from build123d import *

# Parameters (mm, degrees)
CROQUIS3_W              = 30
CROQUIS3_H              = 29
SALIENTE_EXTRUIR1_DEPTH = 5
CROQUIS5_W              = 30
CROQUIS5_H              = 29
CROQUIS5_W_2            = 25.5
CROQUIS5_H_2            = 24.5
CORTAR_EXTRUIR1_DEPTH   = 2
CROQUIS9_W              = 25.5
CROQUIS9_H              = 2.25
SALIENTE_EXTRUIR2_DEPTH = 13.5
CROQUIS11_W             = 22
CROQUIS11_H             = 6
CORTAR_EXTRUIR3_DEPTH   = 3
CROQUIS12_W             = 25.5
CROQUIS12_H             = 3.5
SALIENTE_EXTRUIR3_DEPTH = 15
CROQUIS13_W             = 25.5
CROQUIS13_H             = 4
SALIENTE_EXTRUIR4_DEPTH = 20
REDONDEO3_R             = 5
CROQUIS14_R             = 1.5
CORTAR_EXTRUIR4_DEPTH   = 7
REDONDEO5_R             = 10
REDONDEO6_R             = 40
CROQUIS6_R              = 1
CORTAR_EXTRUIR5_DEPTH   = 5
CORTAR_EXTRUIR7_DEPTH   = 2
CROQUIS16_W             = 21.5
CROQUIS16_H             = 5
CORTAR_EXTRUIR8_DEPTH   = 2


with BuildPart() as part:
    # Croquis3 → Saliente-Extruir1 (new body)
    with BuildSketch(Plane.XY):
        Rectangle(CROQUIS3_W, CROQUIS3_H)
    extrude(amount=SALIENTE_EXTRUIR1_DEPTH)

    # Croquis5 → Cortar-Extruir1 (cut)
    with BuildSketch(Plane.XY.offset(5)):
        Rectangle(CROQUIS5_W, CROQUIS5_H)
        Rectangle(CROQUIS5_W_2, CROQUIS5_H_2, mode=Mode.SUBTRACT)
    extrude(amount=-CORTAR_EXTRUIR1_DEPTH, mode=Mode.SUBTRACT)

    # Croquis9 → Saliente-Extruir2 (add)
    with BuildSketch(Plane.XY.offset(3)):
        with Locations((0, -13.375)):
            Rectangle(CROQUIS9_W, CROQUIS9_H)
    extrude(amount=SALIENTE_EXTRUIR2_DEPTH)

    # Croquis11 → Cortar-Extruir3 (cut)
    with BuildSketch(Plane.XZ.offset(14.5)):
        with Locations((0, 7.6)):
            Rectangle(CROQUIS11_W, CROQUIS11_H)
    extrude(amount=-CORTAR_EXTRUIR3_DEPTH, mode=Mode.SUBTRACT)

    # Croquis12 → Saliente-Extruir3 (add)
    with BuildSketch(Plane.XZ.offset(14.5)):
        with Locations((0, 12.75)):
            Rectangle(CROQUIS12_W, CROQUIS12_H)
    extrude(amount=SALIENTE_EXTRUIR3_DEPTH)

    # Croquis13 → Saliente-Extruir4 (add)
    with BuildSketch(Plane(origin=(0, 0, 11), x_dir=(-1, 0, 0), z_dir=(0, 0, -1))):
        with Locations((0, -27.5)):
            Rectangle(CROQUIS13_W, CROQUIS13_H)
    extrude(amount=SALIENTE_EXTRUIR4_DEPTH)

    # Redondeo3
    redondeo3_edges = [part.edges().sort_by_distance(p)[0] for p in [
        (0, -29.5, 14.5),
    ]]
    fillet(redondeo3_edges, radius=REDONDEO3_R)

    # Croquis14 → Cortar-Extruir4 (cut)
    with BuildSketch(Plane.XZ.offset(29.5)):
        with Locations((0, -3)):
            Circle(CROQUIS14_R)
    extrude(amount=-CORTAR_EXTRUIR4_DEPTH, mode=Mode.SUBTRACT)

    # Redondeo5
    # the kernel refuses this fillet: 10 mm, written as the material it adds along each edge
    with BuildSketch(Plane(origin=(12.75, -14.5, 11), x_dir=(0, -1, 0), z_dir=(-1, 0, 0))) as redondeo5_piece_1_section:
        with BuildLine():
            CenterArc((REDONDEO5_R, -REDONDEO5_R), REDONDEO5_R, 90, 90)
            Line((0, -REDONDEO5_R), (0, 0))
            Line((0, 0), (REDONDEO5_R, 0))
        make_face()
    redondeo5_piece_1 = extrude(amount=50.5, mode=Mode.PRIVATE)
    redondeo5_piece_1 = split(redondeo5_piece_1, bisect_by=Plane(origin=(11, -14.5, 11), z_dir=(1, 0, 0)), keep=Keep.TOP, mode=Mode.PRIVATE)
    add(redondeo5_piece_1)
    with BuildSketch(Plane(origin=(37.75, -14.5, 11), x_dir=(0, -1, 0), z_dir=(-1, 0, 0))) as redondeo5_piece_2_section:
        with BuildLine():
            CenterArc((REDONDEO5_R, -REDONDEO5_R), REDONDEO5_R, 90, 90)
            Line((0, -REDONDEO5_R), (0, 0))
            Line((0, 0), (REDONDEO5_R, 0))
        make_face()
    redondeo5_piece_2 = extrude(amount=50.5, mode=Mode.PRIVATE)
    redondeo5_piece_2 = split(redondeo5_piece_2, bisect_by=Plane(origin=(11, -14.5, 11), z_dir=(-1, 0, 0)), keep=Keep.TOP, mode=Mode.PRIVATE)
    redondeo5_piece_2 = split(redondeo5_piece_2, bisect_by=Plane(origin=(37.75, -14.5, 10.6), z_dir=(0, 0, 1)), keep=Keep.TOP, mode=Mode.PRIVATE)
    add(redondeo5_piece_2)
    with BuildSketch(Plane(origin=(37.75, -14.5, 11), x_dir=(0, -1, 0), z_dir=(-1, 0, 0))) as redondeo5_piece_3_section:
        with BuildLine():
            CenterArc((REDONDEO5_R, -REDONDEO5_R), REDONDEO5_R, 90, 90)
            Line((0, -REDONDEO5_R), (0, 0))
            Line((0, 0), (REDONDEO5_R, 0))
        make_face()
    redondeo5_piece_3 = extrude(amount=75.5, mode=Mode.PRIVATE)
    redondeo5_piece_3 = split(redondeo5_piece_3, bisect_by=Plane(origin=(37.75, -14.5, 3), z_dir=(0, 0, -1)), keep=Keep.TOP, mode=Mode.PRIVATE)
    redondeo5_piece_3 = split(redondeo5_piece_3, bisect_by=Plane(origin=(15, -14.5, 11), z_dir=(-1, 0, 0)), keep=Keep.TOP, mode=Mode.PRIVATE)
    redondeo5_piece_3 = split(redondeo5_piece_3, bisect_by=Plane(origin=(-15, -14.5, 11), z_dir=(1, 0, 0)), keep=Keep.TOP, mode=Mode.PRIVATE)
    add(redondeo5_piece_3)
    with BuildSketch(Plane(origin=(37.75, -14.5, 11), x_dir=(0, -1, 0), z_dir=(-1, 0, 0))) as redondeo5_piece_4_section:
        with BuildLine():
            CenterArc((REDONDEO5_R, -REDONDEO5_R), REDONDEO5_R, 90, 90)
            Line((0, -REDONDEO5_R), (0, 0))
            Line((0, 0), (REDONDEO5_R, 0))
        make_face()
    redondeo5_piece_4 = extrude(amount=50.5, mode=Mode.PRIVATE)
    redondeo5_piece_4 = split(redondeo5_piece_4, bisect_by=Plane(origin=(11, -14.5, 11), z_dir=(-1, 0, 0)), keep=Keep.TOP, mode=Mode.PRIVATE)
    redondeo5_piece_4 = split(redondeo5_piece_4, bisect_by=Plane(origin=(37.75, -14.5, 4.6), z_dir=(0, 0, -1)), keep=Keep.TOP, mode=Mode.PRIVATE)
    add(redondeo5_piece_4)
    with BuildSketch(Plane(origin=(37.75, -14.5, 11), x_dir=(0, -1, 0), z_dir=(-1, 0, 0))) as redondeo5_piece_5_section:
        with BuildLine():
            CenterArc((REDONDEO5_R, -REDONDEO5_R), REDONDEO5_R, 90, 90)
            Line((0, -REDONDEO5_R), (0, 0))
            Line((0, 0), (REDONDEO5_R, 0))
        make_face()
    redondeo5_piece_5 = extrude(amount=50.5, mode=Mode.PRIVATE)
    redondeo5_piece_5 = split(redondeo5_piece_5, bisect_by=Plane(origin=(-11, -14.5, 11), z_dir=(-1, 0, 0)), keep=Keep.TOP, mode=Mode.PRIVATE)
    add(redondeo5_piece_5)
    with BuildSketch(Plane(origin=(-12.75, -14.5, 14.5), x_dir=(0, -1, 0), z_dir=(1, 0, 0))) as redondeo5_piece_6:
        with BuildLine():
            CenterArc((6, -10), REDONDEO5_R, 90, 36.869897646)
            Line((0, -2), (0, 0))
            Line((0, 0), (6, 0))
        make_face()
    extrude(amount=25.5)

    # Redondeo6
    # the kernel refuses this fillet: 40 mm, written as the material it adds along each edge
    with BuildSketch(Plane(origin=(-12.75, -25.5, 11), x_dir=(0, 1, 0), z_dir=(1, 0, 0))) as redondeo6_piece_1:
        with BuildLine():
            CenterArc((40, -8.888194417), REDONDEO6_R, 167.161431859, 12.838568141)
            Line((0, -8.888194417), (-0.8, -8.888194417))
            Line((-0.8, -8.888194417), (-0.8, 0))
            Line((-0.8, 0), (0, 0.8))
            ThreePointArc((0, 0.8), (0.5, 0.8), (0.22, 0.177763888))
            Line((0.22, 0.177763888), (1, 0))
        make_face()
    extrude(amount=25.5)

    # Croquis6 → Cortar-Extruir5 (cut)
    with BuildSketch(Plane.XY):
        with Locations((-10.75, 9.75)):
            Circle(CROQUIS6_R)
        with Locations((-10.75, -3.75)):
            Circle(CROQUIS6_R)
        with Locations(Location((10.75, -3.75, 0), (0, 0, 180))):
            Circle(CROQUIS6_R)
        with Locations(Location((10.75, 9.75, 0), (0, 0, 180))):
            Circle(CROQUIS6_R)
    extrude(amount=CORTAR_EXTRUIR5_DEPTH, mode=Mode.SUBTRACT)

    # Croquis15 → Cortar-Extruir7 (cut)
    with BuildSketch(Plane(origin=(0, 0, 0), x_dir=(-1, 0, 0), z_dir=(0, 0, -1))):
        Polygon((-10.75, 12.636751346), (-13.25, 11.193375673), (-13.25, 8.306624327), (-10.75, 6.863248654), (-8.25, 8.306624327), (-8.25, 11.193375673), align=None)
        Polygon((10.75, 12.636751346), (8.25, 11.193375673), (8.25, 8.306624327), (10.75, 6.863248654), (13.25, 8.306624327), (13.25, 11.193375673), align=None)
        Polygon((10.75, -0.863248654), (8.25, -2.306624327), (8.25, -5.193375673), (10.75, -6.636751346), (13.25, -5.193375673), (13.25, -2.306624327), align=None)
        Polygon((-10.75, -0.863248654), (-13.25, -2.306624327), (-13.25, -5.193375673), (-10.75, -6.636751346), (-8.25, -5.193375673), (-8.25, -2.306624327), align=None)
    extrude(amount=-CORTAR_EXTRUIR7_DEPTH, mode=Mode.SUBTRACT)

    # Croquis16 → Cortar-Extruir8 (cut)
    with BuildSketch(Plane.XY.offset(5)):
        with Locations((0, 3)):
            Rectangle(CROQUIS16_W, CROQUIS16_H)
    extrude(amount=-CORTAR_EXTRUIR8_DEPTH, mode=Mode.SUBTRACT)


solid = part.part
The model under review builds one solid part; all positions refer to its coordinate system, in mm. A direction names the side the tool comes from. Give positions to 0.01 mm unless a question says otherwise; leave off trailing zeros. Loops run counter-clockwise (first coordinate to the right, second up) from the corner with the lowest first, then second, coordinate; pieces in that order, holes last. Notation, with made-up numbers: (23, -26.75) -> (37, -26.75) arc R11 cw to (37, -7.75) -> close; hole circle Ø11 at (30.5, -4). An arc over 180 degrees is marked (long way). Put each result on its own line as item: value. Start each with the question number.
1. We need section A-A on x = 4.5. State the section outline as (y, z) points.
2. Mouldability with a two-part tool opening along Z and no side actions: class faces 1 (the face through (0, -13, 16.5)), 2 (the face through (0, 0, 0)), 3 (the face through (-12.018, 11.905, 0.986)), 4 (the face through (0, -13, 4.6)) as released by +Z, released by -Z, zero draft, split by the parting line, or undercut.
3. Wall thickness on probe 1 along X at (y, z) = (-3.75, 3.8); probe 2 along X at (y, z) = (9.75, 2.7); probe 3 along X at (y, z) = (-17.5, 10.25): over which ranges is each line inside the solid? List them lowest first.
4. We need section D-D on z = 11.75. State the section outline as (x, y) points.
5. For faces 5 (the face through (-8.25, -4, 1)), 6 (the face through (0, 3, 3)), 7 (the face through (0, -17, 10.6)), 8 (the face through (2, 13, 3)), list the 3-axis set-ups (+Z, -Z, +X, -X, +Y, -Y) from which the entire face can be reached by the end or side of a thin tool; tool diameter is ignored.
6. We need section B-B on y = 4.5. State the section outline as (x, z) points.
7. Clearance check with flat-ended pins moving along their axes: P1, Ø0.6, axis at y = 2.5, z = 4.5, coming from the +X side; P2, Ø1.5, axis at x = 10.5, y = 10, coming from the -Z side; P3, Ø3, axis at x = 0.5, y = -18.5, coming from the -Z side; P4, Ø6, axis at y = -21, z = -6, coming from the +X side. State where each tip first meets the part, or that it passes through.
8. We need section C-C on y = -3.75. State the section outline as (x, z) points, then the cut area to 3 significant figures.
Determined:
1. outline: (-29.5, -9) -> (-25.5, -9) -> (-25.5, 2.11) arc R40 cw to (-24.5, 11) arc R10 cw to (-21.7, 10.6) -> (-12.25, 10.6) -> (-12.25, 16.5) -> (-14.5, 16.5) arc R10 cw to (-20.5, 14.5) -> (-24.5, 14.5) arc R5 ccw to (-29.5, 9.5) -> close; (-15.17, 4.6) arc R10 cw to (-14.5, 1) -> (-14.5, 0) -> (14.5, 0) -> (14.5, 3) -> (12.25, 3) -> (12.25, 5) -> (5.5, 5) -> (5.5, 3) -> (0.5, 3) -> (0.5, 5) -> (-11.5, 5) -> (-11.5, 4.6) -> close
2. face 1: released by +Z
2. face 2: released by -Z
2. face 3: zero draft
2. face 4: undercut
3. probe 1: -12.75 to -11.75, -9.75 to 9.75, 11.75 to 12.75
3. probe 2: -15 to -11.75, -9.75 to 9.75, 11.75 to 15
3. probe 3: -12.75 to -11, 11 to 12.75
4. outline: (-12.75, -28.97) -> (12.75, -28.97) -> (12.75, -12.25) -> (-12.75, -12.25) -> close
5. face 5: -Z
5. face 6: +Z
5. face 7: +Y
5. face 8: +Z, +Y
6. outline: (-15, 0) -> (15, 0) -> (15, 3) -> (12.75, 3) -> (12.75, 5) -> (10.75, 5) -> (10.75, 3) -> (-10.75, 3) -> (-10.75, 5) -> (-12.75, 5) -> (-12.75, 3) -> (-15, 3) -> close
7. P1: x = 12.75
7. P2: z = 2
7. P3: z = 10.6
7. P4: through
8. outline: (-15, 0) -> (-13.25, 0) -> (-13.25, 2) -> (-11.75, 2) -> (-11.75, 5) -> (-12.75, 5) -> (-12.75, 3) -> (-15, 3) -> close; (-9.75, 2) -> (-8.25, 2) -> (-8.25, 0) -> (8.25, 0) -> (8.25, 2) -> (9.75, 2) -> (9.75, 5) -> (-9.75, 5) -> close; (11.75, 2) -> (13.25, 2) -> (13.25, 0) -> (15, 0) -> (15, 3) -> (12.75, 3) -> (12.75, 5) -> (11.75, 5) -> close
8. area: 109 mm^2
